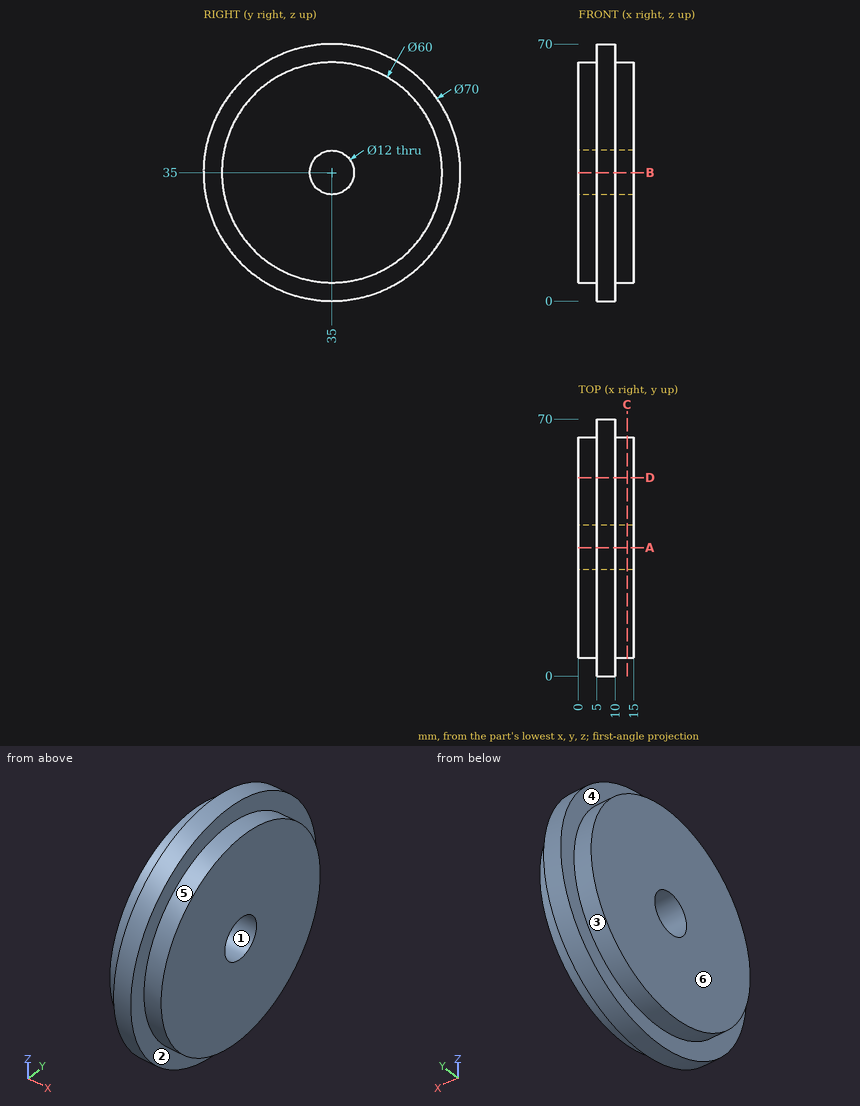
Study the drawing (mm; zero at the part's minimum x, y, z) and answer. A direction names the side the tool comes from. Give positions to 0.01 mm unless a question says otherwise; leave off trailing zeros. Write each loop counter-clockwise with the first axis right and the second up, starting at its lowest first coordinate (ties: lowest second). Pieces come first, ordered by that corner, then holes. Notation, with made-up numbers: (-36.75, 3) - (-12.75, 3) arc R23 ccw to (-12.75, 30) - close; hole circle Ø11 at (29.5, -38). An arc over 180 degrees is marked (long way). Use a Markdown table: item, result.
1. For a pull along Z with two mould halves and no side action, classify the marked faces 1, 2 and 3 as released by +Z, released by -Z, zero draft, split by the parting line, or undercut.
Values follow:
| item | result |
|---|---|
| face 1 | undercut |
| face 2 | zero draft |
| face 3 | split by the parting line |
2. Section D-D on y = 54 is taken. Write down the section's boundary in (x, z).
Values follow:
| item | result |
|---|---|
| outline | (0, 11.78) - (5, 11.78) - (5, 5.61) - (10, 5.61) - (10, 11.78) - (15, 11.78) - (15, 58.22) - (10, 58.22) - (10, 64.39) - (5, 64.39) - (5, 58.22) - (0, 58.22) - close |
3. Section A-A on y = 35 is taken. Write down the section's boundary in (x, z).
Values follow:
| item | result |
|---|---|
| outline | (0, 5) - (5, 5) - (5, 0) - (10, 0) - (10, 5) - (15, 5) - (15, 29) - (0, 29) - close; (0, 41) - (15, 41) - (15, 65) - (10, 65) - (10, 70) - (5, 70) - (5, 65) - (0, 65) - close |
4. Each of these flat-tipped pins is pushed along its axis until it touches: P1, Ø4, axis at x = 9, z = 59.5, coming from the +Y side; P2, Ø2, axis at y = 53.5, z = 10, coming from the +X side; P3, Ø4, axis at x = 13, z = 31, coming from the +Y side. Where does it stop, or does it pass through?
Values follow:
| item | result |
|---|---|
| P1 | stops at y = 61.81 |
| P2 | stops at x = 10 |
| P3 | stops at y = 64.93 |
5. Find the intervals of material crossed by probe 1 along Y at (x, z) = (5.75, 35); probe 2 along Y at (x, z) = (3.5, 35); probe 3 along X at (y, z) = (46, 6.5), in increasing order. Write a range as from..to.
Values follow:
| item | result |
|---|---|
| probe 1 | y = 0..29, 41..70 |
| probe 2 | y = 5..29, 41..65 |
| probe 3 | x = 5..10 |
6. A tool of negligible diameter and unlimited length cuts with its end or side. For the marked faces 4, 5 and 6, from which of +Z, -Z, +X, -X, +Y, -Y can it reach the whole face along a straight path? Write none if from no direction.
Values follow:
| item | result |
|---|---|
| face 4 | -X |
| face 5 | +X |
| face 6 | +Z, -Z, -X, +Y, -Y |
7. Section C-C on x = 13.25 is taken. Write down the section's boundary in (y, z), plus the area to 3 significant figures.
Values follow:
| item | result |
|---|---|
| outline | circle Ø60 at (35, 35); hole circle Ø12 at (35, 35) |
| area | 2,710 mm² |
